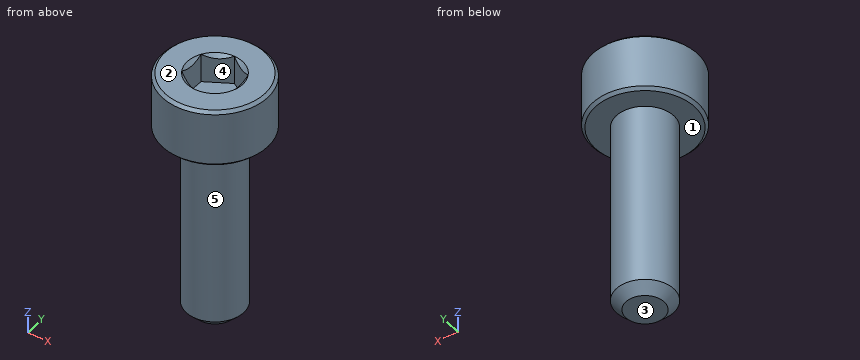
from build123d import *

# Parameters (mm, degrees)
CUT_EXTRUDE1_START = -1.5
CUT_EXTRUDE1_DEPTH = 1.5
SKETCH4_R          = 1.443375673
CUT_EXTRUDE2_DEPTH = 0.5
CUT_EXTRUDE2_TAPER = 45


with BuildPart() as part:
    # Sketch2 → Revolve1 (revolve)
    with BuildSketch(Plane(origin=(0, 0, 0), x_dir=(0, 0, -1), z_dir=(1, 0, 0))):
        Polygon((-6.35, 2.75), (-3.65, 2.75), (-3.5, 2.6), (-3.5, 1.5), (6, 1.5), (6.5, 1), (6.5, 0), (-6.5, 0), (-6.5, 2.6), align=None)
    revolve(axis=Axis((0, 0, -6.5), (0, 0, 1)))

    # Sketch3 → Cut-Extrude1 (cut)
    with BuildSketch(Plane.XY.offset(6.5).offset(CUT_EXTRUDE1_START)):
        Polygon((0, 1.443375673), (-1.25, 0.721687836), (-1.25, -0.721687836), (0, -1.443375673), (1.25, -0.721687836), (1.25, 0.721687836), align=None)
    extrude(amount=CUT_EXTRUDE1_DEPTH, mode=Mode.SUBTRACT)

    # Sketch4 → Cut-Extrude2 (cut)
    with BuildSketch(Plane.XY.offset(6.5)):
        Circle(SKETCH4_R)
    extrude(amount=-CUT_EXTRUDE2_DEPTH, taper=CUT_EXTRUDE2_TAPER, mode=Mode.SUBTRACT)


solid = part.part
Model file for the job. Use its own axes, mm. Face numbers are marked on the shaded views. A direction names the side the tool comes from. Round coordinates to 2 decimals unless told otherwise and drop trailing zeros. Order: outer loops, then holes, each group sorted by start corner. A loop starts at its lowest first (then second) coordinate and runs counter-clockwise, first axis right, second up.
(1) Pull direction Y, two halves, no side cores. Call the marked faces 3, 4 and 5: released by +Y, released by -Y, zero draft, split by the parting line, or undercut.
(2) 3-axis set-ups, long thin cutter, end or side, ignore diameter. For the marked faces 1 and 2: which of +Z, -Z, +X, -X, +Y, -Y reach the whole face in a straight line?
(3) Pin check, flat tips, straight feed: pin 1 (3 mm diameter, centred on y = 2, z = 0, fed in from +X); pin 2 (1.5 mm diameter, centred on y = 1, z = 5, fed in from +X); pin 3 (3 mm diameter, centred on y = -0.5, z = 1, fed in from +X). Stop position of each tip, or through.
(4) Drill centre lines: line 1 (Z direction, x = 0.55, y = 1.6); line 2 (Z direction, x = -0.35, y = -0.3); line 3 (Y direction, x = 0.05, z = -4.75). Where is each one in solid material? Low to high.
(5) Band-saw the part on A-A (y = 0). List the corners of the cut face in (x, z).
(6) Band-saw the part on B-B (z = 0.25). List the corners of the cut face in (x, y).
Verdict:
1. face 3: zero draft
1. face 4: undercut
1. face 5: split by the parting line
2. face 1: -Z
2. face 2: +Z, +X, -X, +Y, -Y
3. pin 1: stops at x = 1.41
3. pin 2: stops at x = 2.74
3. pin 3: stops at x = 1.5
4. line 1: z = 3.5 to 6.5
4. line 2: z = -6.5 to 5
4. line 3: y = -1.5 to 1.5
5. outline: (-2.75, 3.65) - (-2.6, 3.5) - (-1.5, 3.5) - (-1.5, -6) - (-1, -6.5) - (1, -6.5) - (1.5, -6) - (1.5, 3.5) - (2.6, 3.5) - (2.75, 3.65) - (2.75, 6.35) - (2.6, 6.5) - (1.44, 6.5) - (1.25, 6.31) - (1.25, 5) - (-1.25, 5) - (-1.25, 6.31) - (-1.44, 6.5) - (-2.6, 6.5) - (-2.75, 6.35) - close
6. outline: circle Ø3 at (0, 0)
